Work out the finished part from the listing and answer in its coordinate system (mm). A direction names the side the tool comes from. Round coordinates to 2 decimals unless told otherwise and drop trailing zeros. Loops run counter-clockwise (first coordinate to the right, second up) from the corner with the lowest first, then second, coordinate; pieces in that order, holes last. Notation, with made-up numbers: M 30,79 L 70,79 A32 cw 70,105 Z; hole C 78.5,63.5 d4. An arc over 180 degrees is marked long. One line per item, written item: value.
```python
from build123d import *

# Parameters (mm, degrees)
SKETCH1_W               = 8
SKETCH1_H               = 8
BOSS_EXTRUDE1_DEPTH     = 3
CUT_EXTRUDE1_DEPTH      = 12.704699911
CUT_EXTRUDE1_DEPTH_BACK = 12.704699911
CUT_EXTRUDE2_DEPTH      = 11
SKETCH4_R               = 1.8
CUT_EXTRUDE3_DEPTH      = 0.8
SKETCH5_W               = 8
SKETCH5_H               = 1
BOSS_EXTRUDE2_DEPTH     = 2
FILLET1_R               = 4
CUT_EXTRUDE4_DEPTH      = 0.4


with BuildPart() as part:
    # Sketch1 → Boss-Extrude1 (new body)
    with BuildSketch(Plane(origin=(0, 0, 0), x_dir=(1, 0, 0), z_dir=(0, 1, 0))):
        with Locations((4, 4)):
            Rectangle(SKETCH1_W, SKETCH1_H)
    extrude(amount=BOSS_EXTRUDE1_DEPTH)

    # Sketch2 → Cut-Extrude1 (cut, two sides: drawn at the far end of the back side and taken through both)
    with BuildSketch(Plane.XY.offset(-CUT_EXTRUDE1_DEPTH_BACK)):
        Polygon((0, 0), (0.6, 3), (0, 3), align=None)
        Polygon((8, 0), (7.4, 3), (8, 3), align=None)
    extrude(amount=CUT_EXTRUDE1_DEPTH + CUT_EXTRUDE1_DEPTH_BACK, mode=Mode.SUBTRACT)

    # Sketch3 → Cut-Extrude2 (cut)
    with BuildSketch(Plane(origin=(0, 0, 0), x_dir=(0, 0, -1), z_dir=(1, 0, 0))):
        Polygon((0, 0), (0.6, 3), (0, 3), align=None)
        Polygon((8, 3), (7.4, 3), (8, 0), align=None)
    extrude(amount=CUT_EXTRUDE2_DEPTH, mode=Mode.SUBTRACT)

    # Sketch4 → Cut-Extrude3 (cut)
    with BuildSketch(Plane.XZ):
        with Locations(Location((4, -3.75, 0), (0, 0, 270))):
            Circle(SKETCH4_R)
    extrude(amount=-CUT_EXTRUDE3_DEPTH, mode=Mode.SUBTRACT)

    # Sketch5 → Boss-Extrude2 (add)
    with BuildSketch(Plane.XZ):
        with Locations((4, -7.5)):
            Rectangle(SKETCH5_W, SKETCH5_H)
    extrude(amount=BOSS_EXTRUDE2_DEPTH)

    # Fillet1
    # the kernel refuses this fillet: 4 mm, written as the material it takes off along each edge
    with BuildSketch(Plane(origin=(8, -2, -16.660254038), x_dir=(0, 1, 0), z_dir=(0, 0, 1)), Plane(origin=(0, -2, 1.660254038), x_dir=(0, 1, 0), z_dir=(0, 0, -1))) as fillet1_piece_1:
        with BuildLine():
            CenterArc((4, 3.464101615), FILLET1_R, 180, 60)
            Line((0, 3.464101615), (-0.08, 3.464101615))
            Line((-0.08, 3.464101615), (-0.08, 0))
            Line((-0.08, 0), (0, -0.08))
            ThreePointArc((0, -0.08), (1, -0.08), (1.96, -0.069282032))
            Line((1.96, -0.069282032), (2, 0))
        make_face()
    extrude(amount=18.320508076, mode=Mode.SUBTRACT)

    # Sketch6 → Cut-Extrude4 (cut)
    with BuildSketch(Plane(origin=(0, 3, 0), x_dir=(1, 0, 0), z_dir=(0, 1, 0))):
        Polygon((2.358967796, 2.025988971), (1.401435745, 6.025988971), (2.189897284, 6.025988971), (2.811692155, 3.278392817), (3.469544719, 6.025988971), (4.519224207, 6.025988971), (5.170666514, 3.231918458), (5.790858822, 6.025988971), (6.580922925, 6.025988971), (5.641019078, 2.025988971), (4.688294719, 2.025988971), (3.991179335, 5.016373586), (3.275634463, 2.025988971), align=None)
    extrude(amount=-CUT_EXTRUDE4_DEPTH, mode=Mode.SUBTRACT)


solid = part.part
```
1) Find section D-D (y = 2.75). Give the vertices of the cut face in (x, z).
Check values:
outline: M 0.55,-7.45 L 7.45,-7.45 L 7.45,-0.55 L 0.55,-0.55 Z; hole M 1.4,-6.03 L 2.19,-6.03 L 2.81,-3.28 L 3.47,-6.03 L 4.52,-6.03 L 5.17,-3.23 L 5.79,-6.03 L 6.58,-6.03 L 5.64,-2.03 L 4.69,-2.03 L 3.99,-5.02 L 3.28,-2.03 L 2.36,-2.03 Z
2) Each of these flat-tipped pins is pushed along its axis until it touches: pin 1 (2 mm diameter, centred on x = 4.5, y = -1.5, fed in from +Z); pin 2 (1.5 mm diameter, centred on y = 1, z = -6.5, fed in from +X); pin 3 (3 mm diameter, centred on x = 4.5, z = -3.5, fed in from -Y). Where does it stop, or does it pass through?
Check values:
pin 1: z = -7
pin 2: x = 7.95
pin 3: y = 0
3) Find section A-A (y = 0.5). Give the vertices of the cut face in (x, z), then the cut area to 3 significant figures.
Check values:
outline: M 0.1,-7.9 L 7.9,-7.9 L 7.9,-0.1 L 0.1,-0.1 Z; hole C 4,-3.75 d3.6
area: 50.7 mm2
4) For faces 1 (the face through (4, 3, -4)), 2 (the face through (4, 0.8, -4)), 3 (the face through (3.5, 2.6, -4.1)), 4 (the face through (3, 0, -2)), determine the directions among +Z, -Z, +X, -X, +Y, -Y from which every point of the face is accessible in a straight line to the end or side of a thin tool.
Check values:
face 1: +Z, -Z, +X, -X, +Y
face 2: -Y
face 3: +Y
face 4: +Z, +X, -X, -Y
5) The mould has two halves that part along X. Classify faces 5 (the face through (4.541, 0.394, -5.467)), 6 (the face through (6.51, -1.48, -7.51)), 7 (the face through (4, -2, -7.5)): +X half, -X half, draft (parallel to the pull), parting line (faces both ways), or undercut.
Check values:
face 5: undercut
face 6: +X half
face 7: draft
6) Find the intervals of material crossed by probe 1 along Y at (x, z) = (1.25, -6.75); probe 2 along Y at (x, z) = (5.75, -4.5); probe 3 along Z at (x, y) = (1.75, -1.15), in increasing order. Write a range as from..to.
Check values:
probe 1: 0..3
probe 2: 0..2.6
probe 3: -8..-7
7) Find section C-C (x = 3.75). Give the vertices of the cut face in (y, z).
Check values:
outline: M -2,-8 L 0,-8 L 3,-7.4 L 3,-6.03 L 2.6,-6.03 L 2.6,-4.01 L 3,-4.01 L 3,-0.6 L 0,0 L 0,-1.97 L 0.8,-1.97 L 0.8,-5.53 L 0,-5.53 L 0,-7 L -2,-7 Z
8) Find section B-B (z = -2.75). Give the vertices of the cut face in (x, y).
Check values:
outline: M 0,0 L 2.5,0 L 2.5,0.8 L 5.5,0.8 L 5.5,0 L 8,0 L 7.4,3 L 5.81,3 L 5.81,2.6 L 4.52,2.6 L 4.52,3 L 3.45,3 L 3.45,2.6 L 2.19,2.6 L 2.19,3 L 0.6,3 Z
